```python
from build123d import *

# Parameters (mm, degrees)
SKETCH1_R           = 5.775
BOSS_EXTRUDE1_DEPTH = 4.5
BOSS_EXTRUDE1_TAPER = 2
SKETCH2_R           = 4
BOSS_EXTRUDE2_DEPTH = 5.15
FILLET1_R           = 0.5
FILLET2_R           = 0.25
CUT_EXTRUDE1_START  = -0.1
SKETCH3_R           = 5.13501215
SKETCH3_R_2         = 4
CUT_EXTRUDE1_DEPTH  = 0.1
CUT_EXTRUDE2_DEPTH  = 0.1
SKETCH5_W           = 5.187150014
SKETCH5_H           = 0.489897502
CUT_EXTRUDE3_DEPTH  = 0.1


with BuildPart() as part:
    # Sketch1 → Boss-Extrude1 (new body)
    with BuildSketch(Plane(origin=(0, 0, 0), x_dir=(0, 0, -1), z_dir=(1, 0, 0))):
        Circle(SKETCH1_R)
    extrude(amount=BOSS_EXTRUDE1_DEPTH, taper=BOSS_EXTRUDE1_TAPER)

    # Sketch2 → Boss-Extrude2 (add)
    with BuildSketch(Plane.ZY):
        Circle(SKETCH2_R)
    extrude(amount=-BOSS_EXTRUDE2_DEPTH)

    # Fillet1
    fillet1_edges = [part.edges().sort_by_distance(p)[0] for p in [
        (4.5, 0, 5.617856537),
    ]]
    fillet(fillet1_edges, radius=FILLET1_R)

    # Fillet2
    fillet2_edges = [part.edges().sort_by_distance(p)[0] for p in [
        (5.15, 0, -4),
    ]]
    fillet(fillet2_edges, radius=FILLET2_R)

    # Sketch3 → Cut-Extrude1 (cut)
    with BuildSketch(Plane(origin=(4.5, 0, 0), x_dir=(0, 0, -1), z_dir=(1, 0, 0)).offset(CUT_EXTRUDE1_START)):
        Circle(SKETCH3_R)
        with Locations(Location((0, 0, 0), (0, 0, 180))):
            Circle(SKETCH3_R_2, mode=Mode.SUBTRACT)
    extrude(amount=CUT_EXTRUDE1_DEPTH, mode=Mode.SUBTRACT)

    # Sketch4 → Cut-Extrude2 (cut)
    with BuildSketch(Plane.ZY):
        Polygon((-0.273766251, -2.535940007), (0.273766251, -2.535940007), (0.273766251, -0.280846858), (2.456875417, -0.280846858), (2.456875417, 0.280846858), (0.273766251, 0.280846858), (0.273766251, 2.535940007), (-0.273766251, 2.535940007), (-0.273766251, 0.280846858), (-2.456875417, 0.280846858), (-2.456875417, -0.280846858), (-0.273766251, -0.280846858), align=None)
    extrude(amount=-CUT_EXTRUDE2_DEPTH, mode=Mode.SUBTRACT)

    # Sketch5 → Cut-Extrude3 (cut)
    with BuildSketch(Plane(origin=(5.15, 0, 0), x_dir=(0, 0, -1), z_dir=(1, 0, 0))):
        Rectangle(SKETCH5_W, SKETCH5_H)
    extrude(amount=-CUT_EXTRUDE3_DEPTH, mode=Mode.SUBTRACT)


solid = part.part
```
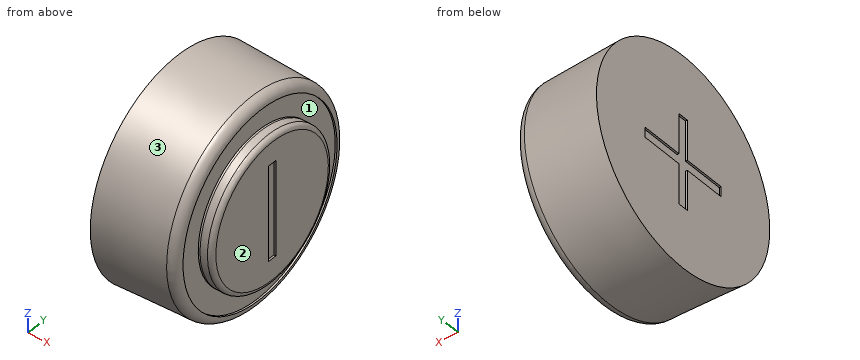
For this review, take the finished solid that the model builds, in its own axes (mm). Face numbers are marked on the shaded views. Coordinates: 2 decimals unless noted, no trailing zeros. Loops run counter-clockwise (first coordinate to the right, second up) from the corner with the lowest first, then second, coordinate; pieces in that order, holes last. Notation, with made-up numbers: (87, 43) - (92, 43) arc R22 cw to (92, 59) - close; hole circle Ø8 at (-27, 72). An arc over 180 degrees is marked (long way). Use one line per item in the form item = value. Start each with the question number.
1) To check wall thickness, follow probe 1 along X at (y, z) = (3, 3); probe 2 along Y at (x, z) = (4.55, 0); probe 3 along Z at (x, y) = (0.6, 2.75). State the ranges of each line that lie inside material, in increasing order. Write a range as from..to.
2) Take a section at B-B (x = 1.55). State the section outline as (y, z) points.
3) Draft analysis for pull direction Z (two halves, no side actions). For the marked faces 1, 2 and 3, state which applies: released by +Z, released by -Z, zero draft, split by the parting line, or undercut.
4) Take a section at C-C (x = 3.1). State the section outline as (y, z) points.
5) For pin 1 (1 mm diameter, centred on x = 3, z = -2, fed in from +Y); pin 2 (2 mm diameter, centred on x = 3, y = 0.5, fed in from +Z); pin 3 (3 mm diameter, centred on x = 2, y = -4.5, fed in from -Z), all flat-tipped, find the tip position at first contact; note any pin that passes through.
6) Take a section at A-A (z = 0). State the section outline as (x, y) points (3 decimals).
From the geometry:
q1.probe_1 = 0..4.4
q1.probe_2 = -4..4
q1.probe_3 = -5.05..5.05
q2.outline = circle Ø11.44 at (0, 0)
q3.face_1 = undercut
q3.face_2 = zero draft
q3.face_3 = split by the parting line
q4.outline = circle Ø11.33 at (0, 0)
q5.pin_1 = 5.47
q5.pin_2 = 5.7
q5.pin_3 = -4.85
q6.outline = (0, -5.775) - (4.017, -5.635) arc R0.5 ccw to (4.5, -5.135) - (4.4, -5.135) - (4.4, -4) - (4.9, -4) arc R0.25 ccw to (5.15, -3.75) - (5.15, -0.245) - (5.05, -0.245) - (5.05, 0.245) - (5.15, 0.245) - (5.15, 3.75) arc R0.25 ccw to (4.9, 4) - (4.4, 4) - (4.4, 5.135) - (4.5, 5.135) arc R0.5 ccw to (4.017, 5.635) - (0, 5.775) - (0, 2.536) - (0.1, 2.536) - (0.1, -2.536) - (0, -2.536) - close
